from build123d import *

# Parameters (mm, degrees)
SKETCH1_W           = 234.19
SKETCH1_H           = 457.2
BOSS_EXTRUDE1_DEPTH = 6.35
SKETCH2_W           = 6.35
SKETCH2_H           = 457.2
BOSS_EXTRUDE2_DEPTH = 457.2
SKETCH3_R           = 14.29
CUT_EXTRUDE1_DEPTH  = 558.8
CUT_EXTRUDE2_DEPTH  = 3.25


with BuildPart() as part:
    # Sketch1 → Boss-Extrude1 (new body)
    with BuildSketch(Plane(origin=(0, 0, 0), x_dir=(1, 0, 0), z_dir=(0, 1, 0))):
        Rectangle(SKETCH1_W, SKETCH1_H)
    extrude(amount=-BOSS_EXTRUDE1_DEPTH)

    # Sketch2 → Boss-Extrude2 (add)
    with BuildSketch(Plane.XZ.offset(6.35)):
        with Locations((-113.92, 0)):
            Rectangle(SKETCH2_W, SKETCH2_H)
    boss_extrude2 = extrude(amount=BOSS_EXTRUDE2_DEPTH)

    # Mirror1: Boss-Extrude2 across plane
    add(boss_extrude2.mirror(Plane(origin=(0, 0, 0), x_dir=(0, 0, 1), z_dir=(1, 0, 0))))

    # Sketch3 → Cut-Extrude1 (cut)
    with BuildSketch(Plane(origin=(117.095, 0, 0), x_dir=(0, 0, -1), z_dir=(1, 0, 0))):
        with Locations((0, -418.55)):
            Circle(SKETCH3_R)
    extrude(amount=-CUT_EXTRUDE1_DEPTH, mode=Mode.SUBTRACT)

    # Sketch4 → Cut-Extrude2 (cut)
    with BuildSketch(Plane(origin=(0, 0, 0), x_dir=(1, 0, 0), z_dir=(0, 1, 0))):
        with BuildLine():
            Line((9.013878189, 3), (12, 3))
            Line((12, 3), (12, -3))
            Line((12, -3), (9.013878189, -3))
            ThreePointArc((9.013878189, -3), (-9.5, 0), (9.013878189, 3))
        make_face()
    extrude(amount=-CUT_EXTRUDE2_DEPTH, mode=Mode.SUBTRACT)


solid = part.part
Could you check a few things on this model? Use its own coordinates, in mm. A direction names the side the tool comes from. Coordinates: 2 decimals unless noted, no trailing zeros. Order: outer loops, then holes, each group sorted by start corner. A loop starts at its lowest first (then second) coordinate and runs counter-clockwise, first axis right, second up.
Q1. Please list where these lines run through material, in increasing order: L1, parallel to Z at x = 0, y = -2.15; L2, parallel to X at y = -64.5, z = 7 (3 decimals); L3, parallel to Y at x = 115.5, z = 0.
Q2. Will these pins go through, and if not, where does the flat tip stop? pin 1 (4 mm diameter, centred on x = -92, z = -118.5, fed in from -Y); pin 2 (15 mm diameter, centred on x = 0, z = 0, fed in from +Y).
Q3. Suppose I cut it at B-B on z = -67.5. Please give me the cut outline in (x, y) (3 decimals), and give its area (3 significant figures).
Q4. Suppose I cut it at A-A on y = -418.55. Please give me the cut outline in (x, z) (3 decimals), and give its area (3 significant figures).
Q5. Which directions (+Z, -Z, +X, -X, +Y, -Y) give clear straight access to the entire face, cutting with the end or side of a thin tool? Please do faces 4 (the cylindrical face through (-9.493, -1.602, 0.375)), 5 (the flat face through (117.095, -229, -3)), 6 (the flat face through (-110.745, -232, -3)).
Q6. Suppose I cut it at C-C on x = 0. Please give me the cut outline in (y, z), and give its area (3 significant figures).
Q7. Thinking about a two-plate mould opening in Y: for faces 1 (the flat face through (110.745, -232, -3)), 2 (the flat face through (24, 0, -3)), 3 (the cylindrical face through (-113.9, -432.5, 3.1)), which applies, released by +Y, released by -Y, zero draft, split by the parting line, or undercut?
Answer:
1. L1: z = -228.6 to -9.5, 9.5 to 228.6
1. L2: x = -117.095 to -110.745, 110.745 to 117.095
1. L3: y = -463.55 to -432.84, -404.26 to 0
2. pin 1: stops at y = -6.35
2. pin 2: stops at y = -3.25
3. outline: (-117.095, -463.55) - (-110.745, -463.55) - (-110.745, -6.35) - (110.745, -6.35) - (110.745, -463.55) - (117.095, -463.55) - (117.095, 0) - (-117.095, 0) - close
3. area: 7,290 mm2
4. outline: (-117.095, -228.6) - (-110.745, -228.6) - (-110.745, -14.29) - (-117.095, -14.29) - close; (-117.095, 14.29) - (-110.745, 14.29) - (-110.745, 228.6) - (-117.095, 228.6) - close; (110.745, -228.6) - (117.095, -228.6) - (117.095, -14.29) - (110.745, -14.29) - close; (110.745, 14.29) - (117.095, 14.29) - (117.095, 228.6) - (110.745, 228.6) - close
4. area: 5,440 mm2
5. face 4: +Y
5. face 5: +Z, -Z, +X, +Y, -Y
5. face 6: +Z, -Z, -Y
6. outline: (-6.35, -228.6) - (0, -228.6) - (0, -9.5) - (-3.25, -9.5) - (-3.25, 9.5) - (0, 9.5) - (0, 228.6) - (-6.35, 228.6) - close
6. area: 2,840 mm2
7. face 1: zero draft
7. face 2: released by +Y
7. face 3: undercut
